Work out the finished part from the listing and answer in its coordinate system (mm). A direction names the side the tool comes from. Give positions to 0.01 mm unless a question says otherwise; leave off trailing zeros. Write each loop counter-clockwise with the first axis right and the second up, starting at its lowest first coordinate (ties: lowest second). Pieces come first, ordered by that corner, then holes. Notation, with made-up numbers: (68.5, 38) -> (107.5, 38) arc R14 ccw to (107.5, 59) -> close; hole circle Ø6 at (1.5, 64.5). An arc over 180 degrees is marked (long way). Use a Markdown table: item, result. Add a question column.
Q1. Section C-C, the plane y = 5 is taken. Give the vertices of the cut face in (x, z), plus the area to 3 significant figures.
Q2. Section B-B, the plane z = -2 is taken. Give the vertices of the cut face in (x, y), plus the area to 3 significant figures.
Q3. For faces 4 (the face through (-5.448, -0.042, 12.665)), 5 (the face through (0, -4.636, -4)), 6 (the face through (-5.5, 3, 0)), 7 (the face through (-3, 4, 19.05)), determine the directions among +Z, -Z, +X, -X, +Y, -Y from which every point of the face is accessible in a straight line to the end or side of a thin tool.
Q4. For a pull along X with two mould halves and no side action, classify faces 1 (the face through (4.03, 2.29, -4)), 2 (the face through (5.944, -0.262, 9.392)), 3 (the face through (-5.5, 0.2, -6.35)) as pulls with the +X half, pulls with the -X half, needs draft (parallel to the pull), parting line crosses it, or undercut.
Q5. Section D-D, the plane z = 8.25 is taken. Give the vertices of the cut face in (x, y), plus the area to 3 significant figures.
Q6. Each of these flat-tipped pins is pushed along its axis until it touches: pin 1 Ø4 at (x, y) = (0, 0) entering from -Z; pin 2 Ø5 at (x, y) = (0, 0) entering from -Z; pin 3 Ø6 at (x, z) = (8, 6) entering from -Y; pin 4 Ø4 at (x, y) = (-8.5, 8.5) entering from +Z. Where does it stop, or does it pass through?
Q7. Section A-A, the plane x = 0 is taken. Give the vertices of the cut face in (y, z).
Q8. Consider line 1 (Y direction, x = 0, z = 13.5); line 2 (Z direction, x = -5, y = -9); line 3 (Y direction, x = 1, z = 5). Determine where each line is inside the solid, lowest interval first.
from build123d import *

# Parameters (mm, degrees)
SKETCH1_R           = 5.95
BOSS_EXTRUDE1_DEPTH = 19.05
SKETCH2_R           = 12.7
BOSS_EXTRUDE2_DEPTH = 6.35
SKETCH3_R           = 4.064
CUT_EXTRUDE1_DEPTH  = 15.875
BOSS_EXTRUDE3_REACH = 25.971
SKETCH7_R           = 4.2164
SKETCH7_R_2         = 4.064
CUT_EXTRUDE2_DEPTH  = 4.7625
MOVE_START          = -6.35
MOVE_FACE1_DEPTH    = 4.7625
SKETCH9_W           = 6
SKETCH9_H           = 6
CUT_EXTRUDE3_DEPTH  = 30.024106225
DRAFT1_ANGLE        = 65


# Read off the part's stored shape, not the designer's step: Move Face1
with BuildPart() as part:
    # Sketch1 → Boss-Extrude1 (new body)
    with BuildSketch(Plane.XY):
        with Locations(Location((0, 0, 0), (0, 0, 180))):
            Circle(SKETCH1_R)
    extrude(amount=BOSS_EXTRUDE1_DEPTH)

    # Sketch2 → Boss-Extrude2 (add)
    with BuildSketch(Plane(origin=(0, 0, 0), x_dir=(-1, 0, 0), z_dir=(0, 0, -1))):
        Circle(SKETCH2_R)
    extrude(amount=BOSS_EXTRUDE2_DEPTH)

    # Sketch3 → Cut-Extrude1 (cut)
    with BuildSketch(Plane.XY.offset(19.05)):
        Circle(SKETCH3_R)
    extrude(amount=-CUT_EXTRUDE1_DEPTH, mode=Mode.SUBTRACT)

    # Sketch6 → CSK for #8 Flat Head Machine Screw (100)1 (revolve, cut)
    with BuildSketch(Plane(origin=(0, 0, 3.175), x_dir=(0, -1, 0), z_dir=(1, 0, 0))):
        Polygon((0, 0), (0, 9.525), (2.2479, 9.525), (2.2479, 1.651767624), (4.2164, 0), align=None)
    revolve(axis=Axis((0, 0, 9.525), (0, 0, -1)), mode=Mode.SUBTRACT)

    # Sketch7 → Boss-Extrude3 (add, up to next)
    with BuildSketch(Plane(origin=(0, 0, 3.175), x_dir=(-1, 0, 0), z_dir=(0, 0, -1)), mode=Mode.PRIVATE) as boss_extrude3_sk1:
        Circle(SKETCH7_R)
        with Locations(Location((0, 0, 0), (0, 0, 180))):
            Circle(SKETCH7_R_2, mode=Mode.SUBTRACT)
    boss_extrude3_tool1 = extrude(boss_extrude3_sk1.sketch, amount=BOSS_EXTRUDE3_REACH, mode=Mode.PRIVATE) - part.part
    add(boss_extrude3_tool1.solids().sort_by_distance((4.097142, 0, 3.175))[0])

    # Sketch8 → Cut-Extrude2 (cut)
    with BuildSketch(Plane(origin=(0, 0, -6.35), x_dir=(-1, 0, 0), z_dir=(0, 0, -1))):
        Polygon((2.529660204, -4.3815), (5.059320409, 0), (2.529660204, 4.3815), (-2.529660204, 4.3815), (-5.059320409, 0), (-2.529660204, -4.3815), align=None)
    extrude(amount=-CUT_EXTRUDE2_DEPTH, mode=Mode.SUBTRACT)

    # Move Face1 outline → Move Face1 (cut)
    with BuildSketch(Plane.XY.offset(MOVE_START)):
        Polygon((-5.352614346, 0), (-2.676307173, -4.6355), (2.676307173, -4.6355), (5.352614346, 0), (2.676307173, 4.6355), (-2.676307173, 4.6355), align=None)
        Polygon((2.529660204, -4.3815), (-2.529660204, -4.3815), (-5.059320409, 0), (-2.529660204, 4.3815), (2.529660204, 4.3815), (5.059320409, 0), align=None, mode=Mode.SUBTRACT)
    extrude(amount=MOVE_FACE1_DEPTH, mode=Mode.SUBTRACT)

    # Sketch9 → Cut-Extrude3 (cut, through all)
    with BuildSketch(Plane.ZY.offset(5.138336307)):
        with Locations((9, 0)):
            Rectangle(SKETCH9_W, SKETCH9_H)
    extrude(amount=CUT_EXTRUDE3_DEPTH, mode=Mode.SUBTRACT)

    # Draft1
    draft1_faces = [part.faces().sort_by_distance(p)[0] for p in [
        (-5.464978006, 0, 12),
        (-5.464978006, 0, 6),
    ]]
    draft(draft1_faces, Plane(origin=(-5.138336307, 0, 0), x_dir=(0, 0, -1), z_dir=(-1, 0, 0)), DRAFT1_ANGLE)


solid = part.part
Result set:
| question | item | result |
|---|---|---|
| 1 | outline | (-11.67, -6.35) -> (11.67, -6.35) -> (11.67, 0) -> (3.23, 0) -> (3.23, 19.05) -> (-3.23, 19.05) -> (-3.23, 0) -> (-11.67, 0) -> close |
| 1 | area | 271 mm2 |
| 2 | outline | circle Ø25.4 at (0, 0); hole (-5.35, 0) -> (-2.68, -4.64) -> (2.68, -4.64) -> (5.35, 0) -> (2.68, 4.64) -> (-2.68, 4.64) -> close |
| 2 | area | 432 mm2 |
| 3 | face 4 | -X, +Y, -Y |
| 3 | face 5 | -Z |
| 3 | face 6 | +Z |
| 3 | face 7 | +Z, +X, -X, +Y, -Y |
| 4 | face 1 | undercut |
| 4 | face 2 | parting line crosses it |
| 4 | face 3 | needs draft |
| 5 | outline | (-5.14, -3) arc R5.95 ccw (long way) to (-5.14, 3) -> close; hole circle Ø8.13 at (0, 0) |
| 5 | area | 56.0 mm2 |
| 6 | pin 1 | passes through |
| 6 | pin 2 | stops at z = -1.59 |
| 6 | pin 3 | stops at y = -3.23 |
| 6 | pin 4 | stops at z = 0 |
| 7 | outline | (-12.7, -6.35) -> (-4.64, -6.35) -> (-4.64, -1.59) -> (-2.25, -1.59) -> (-2.25, 1.52) -> (-4.06, 3.05) -> (-4.06, 19.05) -> (-5.95, 19.05) -> (-5.95, 0) -> (-12.7, 0) -> close; (2.25, -1.59) -> (4.64, -1.59) -> (4.64, -6.35) -> (12.7, -6.35) -> (12.7, 0) -> (5.95, 0) -> (5.95, 19.05) -> (4.06, 19.05) -> (4.06, 3.05) -> (2.25, 1.52) -> close |
| 8 | line 1 | y = -5.95 to -4.06, 4.06 to 5.95 |
| 8 | line 2 | z = -6.35 to 0 |
| 8 | line 3 | y = -5.87 to -3.94, 3.94 to 5.87 |
